```python
from build123d import *

# Parameters (mm, degrees)
F1_DEPTH = 190.5
F3_D     = 114
F4_DEPTH = 2
F5_R     = 5


with BuildPart() as f1:
    # F0 (on Right) → F1 (new body)
    with BuildSketch(Plane.YZ):
        Polygon((-82.545, 368.3), (-101.6, 260.35), (-66.675, 260.35), (-66.675, 368.3), align=None)
        Polygon((-66.675, 260.35), (-31.75, 260.35), (-50.805, 368.3), (-66.675, 368.3), align=None)
        Polygon((-133.35, 0), (0, 0), (0, 260.35), (-31.75, 260.35), (-66.675, 260.35), (-101.6, 260.35), (-133.35, 260.35), align=None)
    extrude(amount=F1_DEPTH)

    # F3 (through all)
    with Locations(Plane.XZ.offset(133.35)):
        with Locations((95.25, 171.45)):
            Hole(F3_D / 2)

    # F2 (on face) → F4 (join)
    with BuildSketch(Plane.XZ.offset(133.35)):
        Polygon((133.25, 76.3), (95.25, 76.3), (57.25, 76.3), (57.25, 32.3), (133.25, 32.3), align=None)
    extrude(amount=-F4_DEPTH)

    # F5
    f5_edges = [f1.edges().sort_by_distance(p)[0] for p in [
        (0, -133.35, 130.175),
        (95.25, -133.35, 260.35),
        (190.5, -133.35, 130.175),
        (95.25, -133.35, 0),
    ]]
    fillet(f5_edges, radius=F5_R)


solid = f1.part
```
Source: CAD feature listing. Evaluate the final solid. Frame: model axes, mm. A direction names the side the tool comes from. Give positions to 0.01 mm unless a question says otherwise; leave off trailing zeros. Order: outer loops, then holes, each group sorted by start corner. A loop starts at its lowest first (then second) coordinate and runs counter-clockwise, first axis right, second up. Notation, with made-up numbers: (-17.75, 28) -> (22.25, 28) arc R18 ccw to (22.25, 54) -> close; hole circle Ø3 at (60.5, 48). An arc over 180 degrees is marked (long way). Use a Markdown table: item, result.
Q1. Section B-B (z = 171.45). Return the cut outline in (x, y), and give its area (3 significant figures).
A:
| item | result |
|---|---|
| outline | (0, -128.35) arc R5 ccw to (5, -133.35) -> (38.25, -133.35) -> (38.25, 0) -> (0, 0) -> close; (152.25, -133.35) -> (185.5, -133.35) arc R5 ccw to (190.5, -128.35) -> (190.5, 0) -> (152.25, 0) -> close |
| area | 10,200 mm^2 |
Q2. Pull-direction query (X, two-part tool) for faces 1 (the face through (0, -65, 146)), 2 (the face through (190.5, -65, 146)), 3 (the face through (42.596, -65.742, 149.619)), 4 (the face through (94, -66, 368.3)); classes: +X half, -X half, draft (parallel to the pull), parting line (faces both ways), or undercut.
A:
| item | result |
|---|---|
| face 1 | -X half |
| face 2 | +X half |
| face 3 | undercut |
| face 4 | draft |
Q3. Material intervals for line 1 (Z direction, x = 95, y = -57); line 2 (X direction, y = -33, z = 171); line 3 (Z direction, x = 84, y = -118), sorted ascending. Write a range as [from, to].
A:
| item | result |
|---|---|
| line 1 | [0, 114.45], [228.45, 368.3] |
| line 2 | [0, 38.25], [152.25, 190.5] |
| line 3 | [0, 115.57], [227.33, 260.35] |
Q4. Section D-D (x = 148). Return the cut outline in (y, z) (3 decimals).
A:
| item | result |
|---|---|
| outline | (-133.35, 5) arc R5 ccw to (-128.35, 0) -> (0, 0) -> (0, 149.853) -> (-133.35, 149.853) -> close; (-133.35, 193.047) -> (0, 193.047) -> (0, 260.35) -> (-31.75, 260.35) -> (-50.805, 368.3) -> (-82.545, 368.3) -> (-101.6, 260.35) -> (-128.35, 260.35) arc R5 ccw to (-133.35, 255.35) -> close |
Q5. Section A-A (x = 95.25). Return the cut outline in (y, z) (3 decimals), and give its area (3 significant figures).
A:
| item | result |
|---|---|
| outline | (-133.35, 5) arc R5 ccw to (-128.35, 0) -> (0, 0) -> (0, 114.45) -> (-133.35, 114.45) -> close; (-133.35, 228.45) -> (0, 228.45) -> (0, 260.35) -> (-31.75, 260.35) -> (-50.805, 368.3) -> (-82.545, 368.3) -> (-101.6, 260.35) -> (-128.35, 260.35) arc R5 ccw to (-133.35, 255.35) -> close |
| area | 25,000 mm^2 |
Q6. First-contact query: P1, Ø9.5, axis at x = 137, y = -19.5, coming from the +Z side; P2, Ø1, axis at x = 120, y = -83, coming from the -Z side. Flat tips, straight axial feed; report the tip coordinate or a pass-through.
A:
| item | result |
|---|---|
| P1 | z = 260.35 |
| P2 | z = 0 |
Q7. Access query for faces 5 (the face through (94, 0, 99)), 6 (the face through (94, -115, 260.35)), 7 (the face through (94, -16, 260.35)). Directions: +Z, -Z, +X, -X, +Y, -Y. A direction counts if a zero-diameter tool reaches every point of the face in a straight line with its end or side. Return the directions, or none.
A:
| item | result |
|---|---|
| face 5 | +Z, -Z, +X, -X, +Y |
| face 6 | +Z, +X, -X, -Y |
| face 7 | +Z, +X, -X, +Y |
Q8. Section C-C (y = -123.5). Return the cut outline in (x, z), and give its area (3 significant figures).
A:
| item | result |
|---|---|
| outline | (0, 0) -> (190.5, 0) -> (190.5, 260.35) -> (0, 260.35) -> close; hole circle Ø114 at (95.25, 171.45) |
| area | 39,400 mm^2 |
